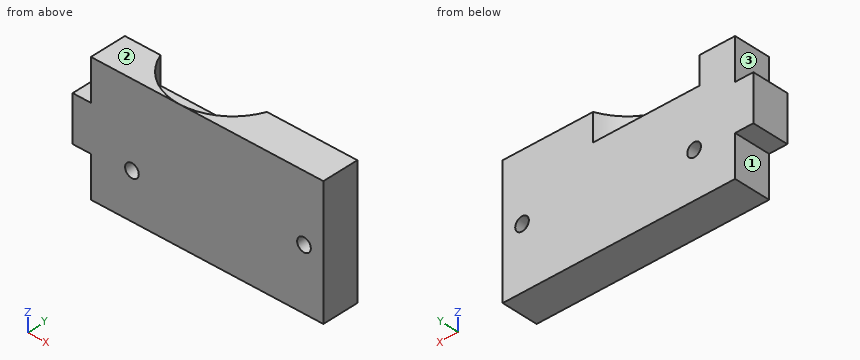
Autodesk Inventor part; units mm, degrees
ref_plane "YZ Plane" through (0, 0, 0) normal (1, 0, 0) x (0, 1, 0)
ref_plane "XZ Plane" through (0, 0, 0) normal (0, 1, 0) x (-1, 0, 0)
ref_plane "XY Plane" through (0, 0, 0) normal (0, 0, 1) x (1, 0, 0)
sketch "Boceto1" plane through (0, 0, 0) normal (0, 1, 0) x (-1, 0, 0)
  line L0 (0, 0) -> (51, 0)
  line L1 (51, 0) -> (51, -28)
  line L2 (51, -28) -> (0, -28)
  line L3 (0, -28) -> (0, 0)
  line L4 (51, 0) -> (51, -18.5)
  line L5 (51, -18.5) -> (42, -18.5)
  circle A0 centre (42, -18.5) radius 1.5
  line L6 (0, 0) -> (0, -14.5)
  line L7 (0, -14.5) -> (4.25, -14.5)
  circle A1 centre (4.25, -14.5) radius 1.5
  line L8 (51, 0) -> (51, -14)
  line L9 (51, -14) -> (55, -14)
  line L10 (55, -14) -> (55, -9)
  line L11 (55, -9) -> (51, -9)
  line L12 (55, -14) -> (55, -19)
  line L13 (55, -19) -> (51, -19)
  dimension "d0" = 51
  dimension "d1" = 28
  dimension "d2" = 18.5
  dimension "d3" = 9
  dimension "d4" = 3
  dimension "d5" = 14.5
  dimension "d6" = 4.25
  dimension "d7" = 3
  dimension "d8" = 14
  dimension "d9" = 4
  dimension "d10" = 5
  dimension "d11" = 5
extrude "Extrusión1" add sketch "Boceto1" along normal blind 2
sketch "Boceto2" plane through (0, 0, 0) normal (0, -1, 0) x (1, 0, 0)
  circle A0 centre (-42, -18.5) radius 1.5
  circle A1 centre (-42, -18.5) radius 1.5
  point P0 (0, 0)
extrude "Extrusión2" add sketch "Boceto2" against normal blind 2
sketch "Boceto3" plane through (0, 0, 0) normal (0, -1, 0) x (1, 0, 0)
  circle A0 centre (-4.25, -14.5) radius 1.5
  circle A1 centre (-4.25, -14.5) radius 1.5
  line L0 (-51, 0) -> (0, 0)
  line L1 (0, 0) -> (-51, 0)
  line L2 (-51, -9) -> (-51, 0)
  line L3 (-51, 0) -> (-51, -9)
  line L4 (-55, -9) -> (-51, -9)
  line L5 (-51, -9) -> (-55, -9)
  line L6 (-51, -19) -> (-55, -19)
  line L7 (-55, -9) -> (-55, -19)
  line L8 (-55, -19) -> (-51, -19)
  line L9 (-51, -28) -> (-51, -19)
  line L10 (-51, -19) -> (-51, -28)
  line L11 (0, -28) -> (-51, -28)
  line L12 (-51, -28) -> (0, -28)
  line L13 (0, 0) -> (0, -28)
  line L14 (0, -28) -> (0, 0)
extrude "Extrusión3" add sketch "Boceto3" along normal blind 6
sketch "Boceto4" plane through (0, -6, 0) normal (0, -1, 0) x (1, 0, 0)
  line L0 (-51, 0) -> (-51, -9)
  line L1 (-51, -9) -> (-51, -18)
  line L2 (-51, -18) -> (-42, -18)
  circle A0 centre (-42, -18) radius 1.5
  point P0 (0, 0)
  dimension "d18" = 9
  dimension "d19" = 9
  dimension "d20" = 3
extrude "Extrusión4" cut sketch "Boceto4" against normal blind 8
sketch "Boceto5" plane through (-51, 2, 0) normal (0, 0, 1) x (1, 0, 0)
  line L0 (51, -8) -> (51, 17)
  line L1 (-4, 4.5) -> (19.5, 4.5)
  circle A0 centre (19.5, 4.5) radius 12.5
  line L2 (0, -8) -> (51, -8)
  line L3 (51, 0) -> (0, 0)
  line L4 (7.8381, 0) -> (31.1619, 0)
  point P0 (51, -2)
  dimension "d23" = 25
  dimension "d24" = 23.5
extrude "Extrusión5" cut sketch "Boceto5" against normal blind 6 contours A0 L3 picked at (19.5, -2.6667)
properties part number "arm_2_microservo_case"
The model under review builds one solid part; all positions refer to its coordinate system, in mm. Face numbers are marked on the shaded views. A direction names the side the tool comes from. Round coordinates to 2 decimals unless told otherwise and drop trailing zeros. Loops run counter-clockwise (first coordinate to the right, second up) from the corner with the lowest first, then second, coordinate; pieces in that order, holes last. Notation, with made-up numbers: M 83,49.25 L 126,49.25 A26 ccw 126,88.25 Z; hole C 35,-2 d3. An arc over 180 degrees is marked long. Answer as a JSON object with one key per item and string values.
Item 1: Tool access review of the marked faces 1, 2 and 3: name each direction out of +Z, -Z, +X, -X, +Y, -Y from which nothing blocks a thin tool from reaching the whole face with its end or side.
Check sheet entries:
{"face 1": "-Z, -X, +Y, -Y", "face 2": "+Z, +X, -X, +Y, -Y", "face 3": "+Z, -X, +Y, -Y"}
Item 2: We need section D-D, the plane x = -41. State the section outline as (y, z) points.
Check sheet entries:
{"outline": "M -6,-28 L 2,-28 L 2,-19.12 L -6,-19.12 Z; M -6,-16.88 L 2,-16.88 L 2,-6 L -1.62,-6 L -1.62,0 L -6,0 Z"}
Item 3: For line 1 along X through (y, z) = (1.5, -14.5); line 2 along Z through (x, y) = (-4.25, -3.6); line 3 along X through (y, z) = (-2.5, -18), list the stretches that pass through material, from the lowest coordinate up.
Check sheet entries:
{"line 1": "-55 to -5.75, -2.75 to 0", "line 2": "-28 to -16, -13 to 0", "line 3": "-55 to -43.5, -40.5 to 0"}
Item 4: We need section A-A, the plane x = -4.25. State the section outline as (y, z) points, and give its area (3 significant figures).
Check sheet entries:
{"outline": "M -6,-28 L 2,-28 L 2,-16 L -6,-16 Z; M -6,-13 L 2,-13 L 2,0 L -6,0 Z", "area": "200 mm2"}
Item 5: Clearance check with flat-ended pins moving along their axes: P1, Ø4.5, axis at x = -53.5, y = -3.5, coming from the +Z side; P2, Ø1, axis at y = -0.5, z = -21.5, coming from the -X side; P3, Ø4, axis at x = -27.5, y = -2, coming from the +Z side. State where each tip first meets the part, or that it passes through.
Check sheet entries:
{"P1": "z = -9", "P2": "x = -51", "P3": "z = -6"}
Item 6: We need section C-C, the plane y = -2.75. State the section outline as (x, z) points.
Check sheet entries:
{"outline": "M -55,-19 L -51,-19 L -51,-28 L 0,-28 L 0,0 L -23.09,0 L -23.09,-6 L -39.91,-6 L -39.91,0 L -51,0 L -51,-9 L -55,-9 Z; hole C -42,-18 d3; hole C -4.25,-14.5 d3"}
